Geometry: final body of the model. Coordinates: model frame, mm. Face numbers are marked on the shaded views. Coordinates: 2 decimals unless noted, no trailing zeros. Loops run counter-clockwise (first coordinate to the right, second up) from the corner with the lowest first, then second, coordinate; pieces in that order, holes last. Notation, with made-up numbers: (69.25, 69.25) -> (105.25, 69.25) arc R19 ccw to (105.25, 91.25) -> close; hole circle Ø2 at (81, -14). An arc over 180 degrees is marked (long way). One line per item, written item: value. Start each with the question number.
Item 1: Contact query for flat-ended pins moving along their axis: pin 1 Ø3 at (y, z) = (-10.5, 1) entering from +X; pin 2 Ø1.5 at (x, z) = (-0.5, 1) entering from -Y; pin 3 Ø1.5 at (y, z) = (-8.5, 1) entering from -X. Output: stop coordinate, or through.
Item 2: Ray query, probe 1 along Y at (x, z) = (0.25, 3.4); probe 2 along Y at (x, z) = (0.5, 1.4); probe 3 along X at (y, z) = (-19.5, 3.2). Return the intervals inside material, ascending. Write a range as from..to.
Item 3: Section query D-D on y = -1. Return loops of the section in (x, z).
Item 4: Section query B-B on z = 2.2. Return loops of the section in (x, y), then the cut area to 3 significant figures.
Item 5: Section query C-C on z = 0.4. Return loops of the section in (x, y).
Item 6: Mould query, pull axis Y, two halves, no side actions, for the marked faces 1, 2 and 3. Classes: +Y half, -Y half, draft (parallel to the pull), parting line (faces both ways), or undercut.
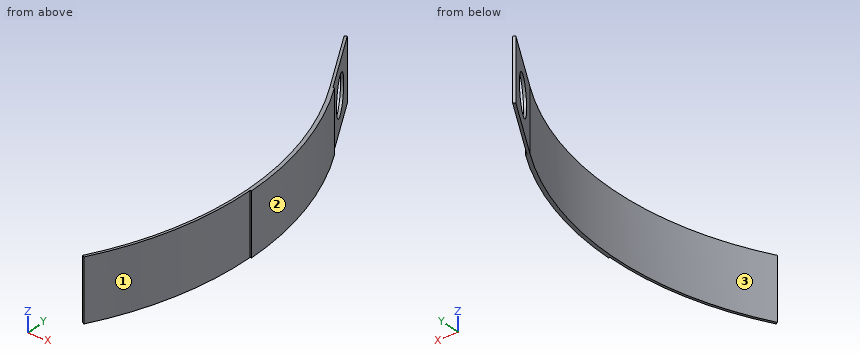
from build123d import *

# Parameters (mm, degrees)
EXTRUDE_1_DEPTH     = 5
SKETCH_2_R          = 1.5
CUT_EXTRUDE_1_DEPTH = 6.698711306
EXTRUDE_2_DEPTH     = 5


with BuildPart() as part:
    # 草图1 → 拉伸-薄壁1 (new body)
    with BuildSketch(Plane.XY):
        with BuildLine():
            ThreePointArc((0, -25), (3.349364905, -12.5), (0, 0))
            Line((0, 0), (-3, 5.196152423))
            Line((-3, 5.196152423), (-3.173205081, 5.096152423))
            Line((-3.173205081, 5.096152423), (-0.173205081, -0.1))
            ThreePointArc((-0.173205081, -0.1), (3.149364905, -12.5), (-0.173205081, -24.9))
            Line((-0.173205081, -24.9), (0, -25))
        make_face()
    extrude(amount=EXTRUDE_1_DEPTH)

    # 草图2 → 切除-拉伸1 (cut, through all)
    with BuildSketch(Plane(origin=(-0.173205081, -0.1, 0), x_dir=(0, 0, 1), z_dir=(-0.866025404, -0.5, 0))):
        with Locations((2.5, 3)):
            Circle(SKETCH_2_R)
    extrude(amount=-CUT_EXTRUDE_1_DEPTH, mode=Mode.SUBTRACT)

    # 草图3 → 拉伸-薄壁2 (add)
    with BuildSketch(Plane.XY):
        with BuildLine():
            ThreePointArc((0, 0), (2.497510563, -6.029523872), (3.349364905, -12.5))
            Line((3.349364905, -12.5), (3.449364905, -12.5))
            ThreePointArc((3.449364905, -12.5), (2.594103145, -6.003641968), (0.08660254, 0.05))
            Line((0.08660254, 0.05), (0, 0))
        make_face()
    extrude(amount=EXTRUDE_2_DEPTH)


solid = part.part
Reply:
1. pin 1: stops at x = 3.44
1. pin 2: stops at y = -25
1. pin 3: stops at x = 2.69
2. probe 1: y = -24.56..-24.14, -0.86..-0.24
2. probe 2: y = -24.09..-23.65, -1.35..-0.69
2. probe 3: x = 2.14..2.35
3. outline: (0.32, 0) -> (0.66, 0) -> (0.66, 5) -> (0.32, 5) -> close
4. outline: (-3.17, 5.1) -> (-2.41, 3.77) -> (-2.23, 3.87) -> (-3, 5.2) -> close; (-0.94, 1.23) -> (-0.17, -0.1) arc R24.8 cw to (-0.17, -24.9) -> (0, -25) arc R25 ccw to (3.35, -12.5) -> (3.45, -12.5) arc R25.1 ccw to (0.09, 0.05) -> (0, 0) -> (-0.77, 1.33) -> close
4. area: 7.14 mm²
5. outline: (-3.17, 5.1) -> (-0.17, -0.1) arc R24.8 cw to (-0.17, -24.9) -> (0, -25) arc R25 ccw to (3.35, -12.5) -> (3.45, -12.5) arc R25.1 ccw to (0.09, 0.05) -> (0, 0) -> (-3, 5.2) -> close
6. face 1: -Y half
6. face 2: +Y half
6. face 3: undercut
